from build123d import *

# Parameters (mm, degrees)
SKETCH1_W           = 210
SKETCH1_H           = 210
BOSS_EXTRUDE1_DEPTH = 3
SKETCH2_W           = 199
SKETCH2_H           = 199
SKETCH2_W_2         = 193
SKETCH2_H_2         = 193
BOSS_EXTRUDE2_DEPTH = 5
SKETCH3_R           = 8
CUT_EXTRUDE1_DEPTH  = 149.707767114
SKETCH5_W           = 52
SKETCH5_H           = 26
SKETCH5_W_2         = 47
SKETCH5_H_2         = 21
BOSS_EXTRUDE4_DEPTH = 6
SKETCH8_W           = 10
SKETCH8_H           = 4
CUT_EXTRUDE2_DEPTH  = 149.707767114
SKETCH9_R           = 5.25
CUT_EXTRUDE3_DEPTH  = 149.707767114


with BuildPart() as part:
    # Sketch1 → Boss-Extrude1 (new body)
    with BuildSketch(Plane(origin=(0, 0, 0), x_dir=(1, 0, 0), z_dir=(0, 1, 0))):
        Rectangle(SKETCH1_W, SKETCH1_H)
    extrude(amount=BOSS_EXTRUDE1_DEPTH)

    # Sketch2 → Boss-Extrude2 (add)
    with BuildSketch(Plane.XZ):
        Rectangle(SKETCH2_W, SKETCH2_H)
        Rectangle(SKETCH2_W_2, SKETCH2_H_2, mode=Mode.SUBTRACT)
    extrude(amount=BOSS_EXTRUDE2_DEPTH)

    # Sketch3 → Cut-Extrude1 (cut, through all)
    with BuildSketch(Plane(origin=(0, 3, 0), x_dir=(1, 0, 0), z_dir=(0, 1, 0))):
        with Locations(Location((-12.805289864, 0, 0), (0, 0, 270))):
            Circle(SKETCH3_R)
        with Locations(Location((12.194710136, 0, 0), (0, 0, 270))):
            Circle(SKETCH3_R)
    extrude(amount=-CUT_EXTRUDE1_DEPTH, mode=Mode.SUBTRACT)

    # Sketch5 → Boss-Extrude4 (add)
    with BuildSketch(Plane(origin=(0, 3, 0), x_dir=(1, 0, 0), z_dir=(0, 1, 0))):
        Rectangle(SKETCH5_W, SKETCH5_H)
        Rectangle(SKETCH5_W_2, SKETCH5_H_2, mode=Mode.SUBTRACT)
    extrude(amount=BOSS_EXTRUDE4_DEPTH)

    # Sketch8 → Cut-Extrude2 (cut, through all)
    with BuildSketch(Plane(origin=(0, 3, 0), x_dir=(1, 0, 0), z_dir=(0, 1, 0))):
        with Locations((0, 17)):
            Rectangle(SKETCH8_W, SKETCH8_H)
    extrude(amount=-CUT_EXTRUDE2_DEPTH, mode=Mode.SUBTRACT)

    # Sketch9 → Cut-Extrude3 (cut, through all)
    with BuildSketch(Plane(origin=(0, 3, 0), x_dir=(1, 0, 0), z_dir=(0, 1, 0))):
        with Locations(Location((-70, 0, 0), (0, 0, 270))):
            Circle(SKETCH9_R)
    extrude(amount=-CUT_EXTRUDE3_DEPTH, mode=Mode.SUBTRACT)


solid = part.part
The model under review builds one solid part; all positions refer to its coordinate system, in mm. A direction names the side the tool comes from. Give positions to 0.01 mm unless a question says otherwise; leave off trailing zeros. Loops run counter-clockwise (first coordinate to the right, second up) from the corner with the lowest first, then second, coordinate; pieces in that order, holes last. Notation, with made-up numbers: (-21.5, 77.25) -> (21.5, 77.25) arc R14 ccw to (21.5, 81.25) -> close; hole circle Ø4 at (88, 62). An arc over 180 degrees is marked (long way). Write each question's results on one line, items separated by ' | '.
1) Draft analysis for pull direction Z (two halves, no side actions). For faces 1 (the face through (-1, -2, 99.5)), 2 (the face through (-1, -2, -96.5)), 3 (the face through (0, 3, 0)), 4 (the face through (-1, 3, -25)), state which applies: pulls with the +Z half, pulls with the -Z half, needs draft (parallel to the pull), parting line crosses it, or undercut.
Conclusion:
face 1: pulls with the +Z half | face 2: undercut | face 3: undercut | face 4: needs draft
2) Insertion check: pin 1 Ø2.5 at (y, z) = (-3, -43.5) entering from -X; pin 2 Ø3 at (x, z) = (-59.5, -45.5) entering from +Y; pin 3 Ø1.8 at (x, y) = (6.5, 6) entering from +Z. Each pin has a flat end and moves straight along its axis. Give the tip position at first contact, or say it passes through.
Conclusion:
pin 1: stops at x = -99.5 | pin 2: stops at y = 3 | pin 3: stops at z = 13
3) Take a section at B-B, the plane y = -2.75. Give the boundary of the cut face in (x, z).
Conclusion:
outline: (-99.5, -99.5) -> (99.5, -99.5) -> (99.5, 99.5) -> (-99.5, 99.5) -> close; hole (-96.5, -96.5) -> (96.5, -96.5) -> (96.5, 96.5) -> (-96.5, 96.5) -> close
4) Tool access review of faces 5 (the face through (99.5, -2, -1)), 6 (the face through (23.5, 6, 0)), 7 (the face through (-26, 6, 0)): name each direction out of +Z, -Z, +X, -X, +Y, -Y from which nothing blocks a thin tool from reaching the whole face with its end or side.
Conclusion:
face 5: +Z, -Z, +X, -Y | face 6: +Y | face 7: +Z, -Z, -X, +Y
5) Take a section at A-A, the plane z = 0. Count the separate pieces of the cut face and the enclosed holes in it, plus the area to 4 significant figures.
Conclusion:
separate pieces: 4 | enclosed holes: 0 | area: 562.5 mm^2
6) Take a section at D-D, the plane z = -69. Give the boundary of the cut face in (x, y).
Conclusion:
outline: (-105, 0) -> (-99.5, 0) -> (-99.5, -5) -> (-96.5, -5) -> (-96.5, 0) -> (96.5, 0) -> (96.5, -5) -> (99.5, -5) -> (99.5, 0) -> (105, 0) -> (105, 3) -> (-105, 3) -> close
7) Take a section at C-C, the plane x = -70. Give the boundary of the cut face in (y, z).
Conclusion:
outline: (-5, -99.5) -> (0, -99.5) -> (0, -105) -> (3, -105) -> (3, -5.25) -> (0, -5.25) -> (0, -96.5) -> (-5, -96.5) -> close; (-5, 96.5) -> (0, 96.5) -> (0, 5.25) -> (3, 5.25) -> (3, 105) -> (0, 105) -> (0, 99.5) -> (-5, 99.5) -> close
8) For line 1 along X through (y, z) = (1.9, 0); line 2 along X through (y, z) = (-3, -57), list the stretches that pass through material, from the lowest coordinate up. Write a range as from..to.
Conclusion:
line 1: x = -105..-75.25, -64.75..-20.81, -4.81..4.19, 20.19..105 | line 2: x = -99.5..-96.5, 96.5..99.5
